Part print with two shaded views. Sizes in mm from the minimum x, y, z corner. Give positions to 0.01 mm unless a question says otherwise; leave off trailing zeros. Loops run counter-clockwise (first coordinate to the right, second up) from the corner with the lowest first, then second, coordinate; pieces in that order, holes last. Notation, with made-up numbers: (80.25, 54) -> (139.25, 54) arc R25 ccw to (139.25, 80) -> close; hole circle Ø9 at (2.5, 9.5). An arc over 180 degrees is marked (long way). One line per question, with ' | ' between items.
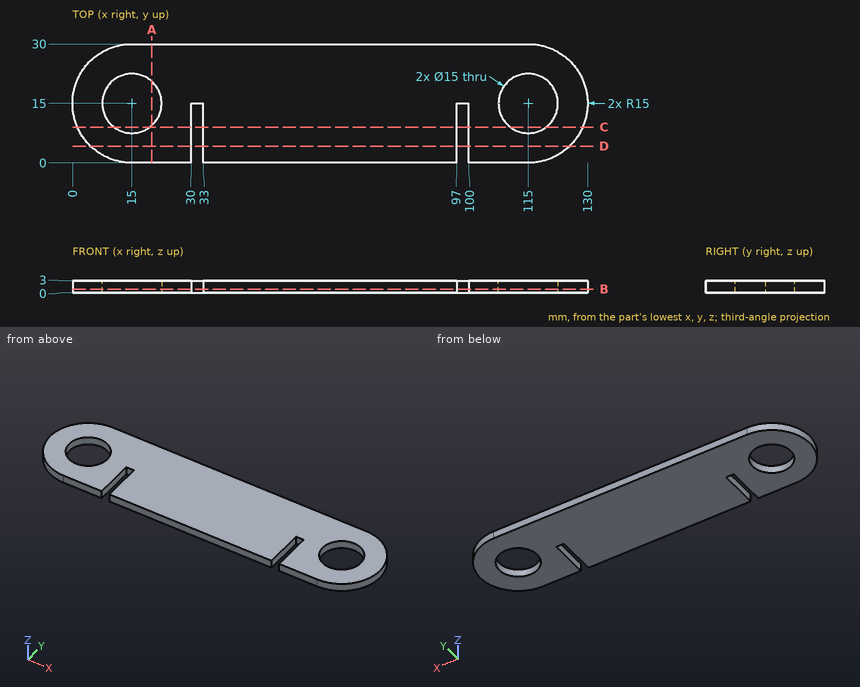
1) Pin check, flat tips, straight feed: P1, Ø1.5, axis at x = 31, z = 1.5, coming from the -Y side; P2, Ø1, axis at y = 18.5, z = 2.5, coming from the -X side; P3, Ø1.5, axis at y = 6.5, z = 2, coming from the -X side. Stop position of each tip, or through.
Found:
P1: y = 15 | P2: x = 0.3 | P3: x = 2.16
2) Saw through at B-B (z = 0.9). Give the cut face in (x, y), and give its area (3 significant figures).
Found:
outline: (15, 0) -> (30, 0) -> (30, 15) -> (33, 15) -> (33, 0) -> (97, 0) -> (97, 15) -> (100, 15) -> (100, 0) -> (115, 0) arc R15 ccw to (115, 30) -> (15, 30) arc R15 ccw to start; hole circle Ø15 at (15, 15); hole circle Ø15 at (115, 15) | area: 3,260 mm2
3) Saw through at C-C (y = 9). Give the cut face in (x, z).
Found:
outline: (1.25, 0) -> (10.5, 0) -> (10.5, 3) -> (1.25, 3) -> close; (19.5, 0) -> (30, 0) -> (30, 3) -> (19.5, 3) -> close; (33, 0) -> (97, 0) -> (97, 3) -> (33, 3) -> close; (100, 0) -> (110.5, 0) -> (110.5, 3) -> (100, 3) -> close; (119.5, 0) -> (128.75, 0) -> (128.75, 3) -> (119.5, 3) -> close
4) Saw through at D-D (y = 4.25). Give the cut face in (x, z), and give its area (3 significant figures).
Found:
outline: (4.54, 0) -> (30, 0) -> (30, 3) -> (4.54, 3) -> close; (33, 0) -> (97, 0) -> (97, 3) -> (33, 3) -> close; (100, 0) -> (125.46, 0) -> (125.46, 3) -> (100, 3) -> close | area: 345 mm2
5) Saw through at A-A (x = 20). Give the cut face in (y, z).
Found:
outline: (0, 0) -> (9.41, 0) -> (9.41, 3) -> (0, 3) -> close; (20.59, 0) -> (30, 0) -> (30, 3) -> (20.59, 3) -> close
6) Drill centre lines: line 1 (X direction, y = 14.75, z = 1.5); line 2 (Y direction, x = 15, z = 2); line 3 (X direction, y = 18, z = 0.2). Where is each one in solid material? Low to high.
Found:
line 1: 0 to 7.5, 22.5 to 30, 33 to 97, 100 to 107.5, 122.5 to 130 | line 2: 0 to 7.5, 22.5 to 30 | line 3: 0.3 to 8.13, 21.87 to 108.13, 121.87 to 129.7
